Could you check a few things on this model? Use its own coordinates, in mm. Face numbers are marked on the shaded views. A direction names the side the tool comes from. Give positions to 0.01 mm unless a question says otherwise; leave off trailing zeros. Order: outer loops, then holes, each group sorted by start corner. A loop starts at its lowest first (then second) coordinate and runs counter-clockwise, first axis right, second up.
from build123d import *

# Parameters (mm, degrees)
SKETCH1_R                      = 29.464
BASE_DEPTH                     = 25.4
FILLET2_R                      = 50.8
BOSS_EXTRUDE3_DEPTH            = 10
MID_FEATURE_BEARING_DEPTH      = 1.524
MID_FEATURE_BEARING_DEPTH_BACK = 1.524
SKETCH8_R                      = 29.464
SKETCH8_R_2                    = 26.924


with BuildPart() as part:
    # Sketch1 → Base (new body)
    with BuildSketch(Plane(origin=(0, 0, 0), x_dir=(1, 0, 0), z_dir=(0, 1, 0))):
        Polygon((-20.613470334, -80.279427719), (20.613470334, -80.279427719), (39.624, 0), (20.613470334, 102.600572281), (-20.613470334, 102.600572281), (-39.624, 0), align=None)
        with Locations(Location((0, 0, 0), (0, 0, 270))):
            Circle(SKETCH1_R, mode=Mode.SUBTRACT)
    extrude(amount=BASE_DEPTH)

    # Fillet2
    fillet2_edges = [part.edges().sort_by_distance(p)[0] for p in [
        (39.624, 12.7, 0),
    ]]
    fillet(fillet2_edges, radius=FILLET2_R)

    # Sketch3 → Boss-Extrude3 (add)
    with BuildSketch(Plane(origin=(0, 25.4, 0), x_dir=(-1, 0, 0), z_dir=(0, -1, 0))):
        with BuildLine():
            Line((51.614471231, 48.928527053), (31.257084114, 45.156572344))
            Line((31.257084114, 45.156572344), (39.624, 0))
            Line((39.624, 0), (32.127488633, -31.65696343))
            Line((32.127488633, -31.65696343), (66.470159483, -25.293720531))
            ThreePointArc((66.470159483, -25.293720531), (67.22595128, -23.21046907), (67.916469509, -21.10468122))
            ThreePointArc((67.916469509, -21.10468122), (64.973148378, -16.061787909), (69.92712938, -12.971159419))
            ThreePointArc((69.92712938, -12.971159419), (70.219719772, -11.280308293), (70.471431194, -9.582890245))
            ThreePointArc((70.471431194, -9.582890245), (69.706370171, -9.476600605), (68.934479365, -9.448308557))
            ThreePointArc((68.934479365, -9.448308557), (65.642119146, -8.297198831), (63.868033442, -5.294315329))
            Line((63.868033442, -5.294315329), (57.38681967, 29.685048936))
            ThreePointArc((57.38681967, 29.685048936), (57.887770412, 32.979114965), (60.322037489, 35.25423396))
            ThreePointArc((60.322037489, 35.25423396), (60.883831005, 35.531602368), (61.420938914, 35.854186128))
            ThreePointArc((61.420938914, 35.854186128), (60.538035517, 37.32560322), (59.61988942, 38.775290915))
            ThreePointArc((59.61988942, 38.775290915), (53.859768583, 39.731805511), (54.646150047, 45.517608517))
            ThreePointArc((54.646150047, 45.517608517), (53.157675832, 47.247390405), (51.614471231, 48.928527053))
        make_face()
        with BuildLine():
            Line((55.84413555, 49.712227935), (51.614471231, 48.928527053))
            ThreePointArc((51.614471231, 48.928527053), (53.157675832, 47.247390405), (54.646150047, 45.517608517))
            ThreePointArc((54.646150047, 45.517608517), (59.06617769, 45.988270979), (61.423391664, 42.219755382))
            ThreePointArc((61.423391664, 42.219755382), (60.945239903, 40.275728903), (59.61988942, 38.775290915))
            ThreePointArc((59.61988942, 38.775290915), (60.538035517, 37.32560322), (61.420938914, 35.854186128))
            ThreePointArc((61.420938914, 35.854186128), (64.301460789, 45.064515776), (55.84413555, 49.712227935))
        make_face()
        with BuildLine():
            ThreePointArc((67.916469509, -21.10468122), (67.22595128, -23.21046907), (66.470159483, -25.293720531))
            Line((66.470159483, -25.293720531), (70.42993181, -24.560027067))
            ThreePointArc((70.42993181, -24.560027067), (76.661646445, -17.088668302), (70.471431194, -9.582890245))
            ThreePointArc((70.471431194, -9.582890245), (70.219719772, -11.280308293), (69.92712938, -12.971159419))
            ThreePointArc((69.92712938, -12.971159419), (72.303225741, -14.435678319), (73.232675696, -17.067554514))
            ThreePointArc((73.232675696, -17.067554514), (71.576309977, -20.405234856), (67.916469509, -21.10468122))
        make_face()
    extrude(amount=BOSS_EXTRUDE3_DEPTH)

    # Sketch8 → mid-feature bearing (add, two sides: drawn at the far end of the back side and taken through both)
    with BuildSketch(Plane(origin=(0, 12.7, 0), x_dir=(1, 0, 0), z_dir=(0, 1, 0)).offset(-MID_FEATURE_BEARING_DEPTH_BACK)):
        with Locations(Location((0, 0, 0), (0, 0, 270))):
            Circle(SKETCH8_R)
        with Locations(Location((0, 0, 0), (0, 0, 270))):
            Circle(SKETCH8_R_2, mode=Mode.SUBTRACT)
    extrude(amount=MID_FEATURE_BEARING_DEPTH + MID_FEATURE_BEARING_DEPTH_BACK)


solid = part.part
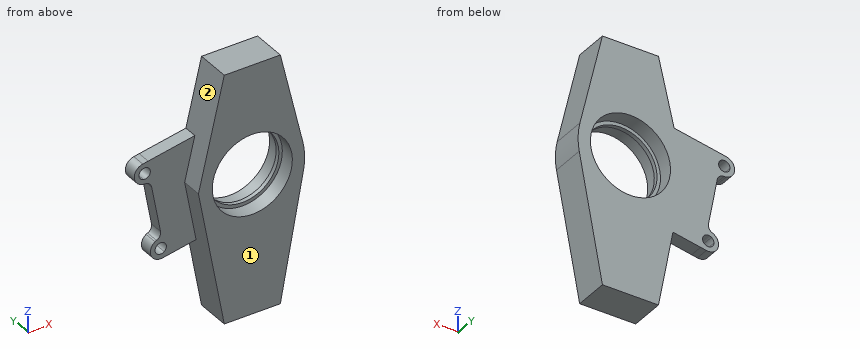
Item 1: Please list where these lines run through material, in increasing order: line 1 along X through (y, z) = (7.5, 0); line 2 along X through (y, z) = (15.5, 14); line 3 along X through (y, z) = (19.5, 0).
Findings:
line 1: x = -39.62 to -29.46, 29.46 to 38.51
line 2: x = -76.02 to -71.9, -66.19 to -25.93, 25.93 to 36.31
line 3: x = -62.89 to -29.46, 29.46 to 38.51
Item 2: Imagine slicing it at C-C on y = 22.5. List the corners of the cut face in (x, z) for me (3 decimals), then the cut area to 3 significant figures.
Findings:
outline: (-70.43, 24.56) arc R7.62 ccw to (-68.934, 9.448) arc R5.08 cw to (-63.868, 5.294) - (-57.387, -29.685) arc R5.08 cw to (-60.322, -35.254) arc R7.62 ccw to (-55.844, -49.712) - (-31.257, -45.157) - (-20.613, -102.601) - (20.613, -102.601) - (37.672, -10.535) arc R50.8 ccw to (37.155, 10.426) - (20.613, 80.279) - (-20.613, 80.279) - (-32.127, 31.657) - close; hole circle Ø8.382 at (-69.042, 17.068); hole circle Ø8.382 at (-57.232, -42.22); hole circle Ø58.928 at (0, 0)
area: 10,400 mm2
Item 3: Imagine slicing it at A-A on x = 0. List the corners of the cut face in (y, z) for me.
Findings:
outline: (0, -102.6) - (25.4, -102.6) - (25.4, -29.46) - (14.22, -29.46) - (14.22, -26.92) - (11.18, -26.92) - (11.18, -29.46) - (0, -29.46) - close; (0, 29.46) - (11.18, 29.46) - (11.18, 26.92) - (14.22, 26.92) - (14.22, 29.46) - (25.4, 29.46) - (25.4, 80.28) - (0, 80.28) - close
Item 4: For the marked faces 1 and 2, which set-ups out of +Z, -Z, +X, -X, +Y, -Y let a thin tool reach every point of the face, with its end or its side?
Findings:
face 1: +Z, -Z, +X, -X, -Y
face 2: +Z, -X, -Y
Item 5: For pin 1 (6 mm diameter, centred on y = 22.5, z = -78, fed in from +X); pin 2 (1 mm diameter, centred on x = -57.5, y = 16.5, fed in from -Z); pin 3 (3 mm diameter, centred on y = 7, z = -32, fed in from +X), each with a flat end and sliding along its axis, tell me the tip position at first contact or that it passes through.
Findings:
pin 1: stops at x = 25.73
pin 2: stops at z = -49.84
pin 3: stops at x = 33.97
Item 6: Imagine slicing it at B-B on y = 3.75. List the corners of the cut face in (x, z) for me (3 decimals), then the cut area to 3 significant figures.
Findings:
outline: (-39.624, 0) - (-20.613, -102.601) - (20.613, -102.601) - (37.672, -10.535) arc R50.8 ccw to (37.155, 10.426) - (20.613, 80.279) - (-20.613, 80.279) - close; hole circle Ø58.928 at (0, 0)
area: 8,280 mm2
Item 7: Imagine slicing it at D-D on z = 61. List the corners of the cut face in (x, y) for me.
Findings:
outline: (-25.18, 0) - (25.18, 0) - (25.18, 25.4) - (-25.18, 25.4) - close
